Part print with two shaded views. Sizes in mm from the minimum x, y, z corner. A direction names the side the tool comes from. Round coordinates to 2 decimals unless told otherwise and drop trailing zeros. Order: outer loops, then holes, each group sorted by start corner. A loop starts at its lowest first (then second) coordinate and runs counter-clockwise, first axis right, second up. Notation, with made-up numbers: (49, -32.75) -> (66, -32.75) arc R9 ccw to (66, -15.75) -> close; hole circle Ø2 at (7.5, 12). An arc over 180 degrees is marked (long way). Use a Markdown table: item, result. Add a question column.
Item 1: Slice it at C-C, the plane x = 76. Give the cut face in (y, z), plus the area to 3 significant figures.
Item 2: Slice it at A-A, the plane z = 130.5. Give the cut face in (x, y).
Item 3: 3-axis set-ups, long thin cutter, end or side, ignore diameter. For the marked faces 5 and 6: which of +Z, -Z, +X, -X, +Y, -Y reach the whole face in a straight line?
Item 4: Slice it at B-B, the plane y = 154.5. Give the cut face in (x, z), plus the area to 3 significant figures.
Item 5: Two-plate mould, pull along X, no slides. Class the marked faces 1, 2, 3 and 4: released by +X, released by -X, zero draft, split by the parting line, or undercut.
Item 6: Probe L1, parallel to X at y = 129.5, z = 51; L2, parallel to Z at x = 222, y = 11. List the from-to ranges inside material, lowest first.
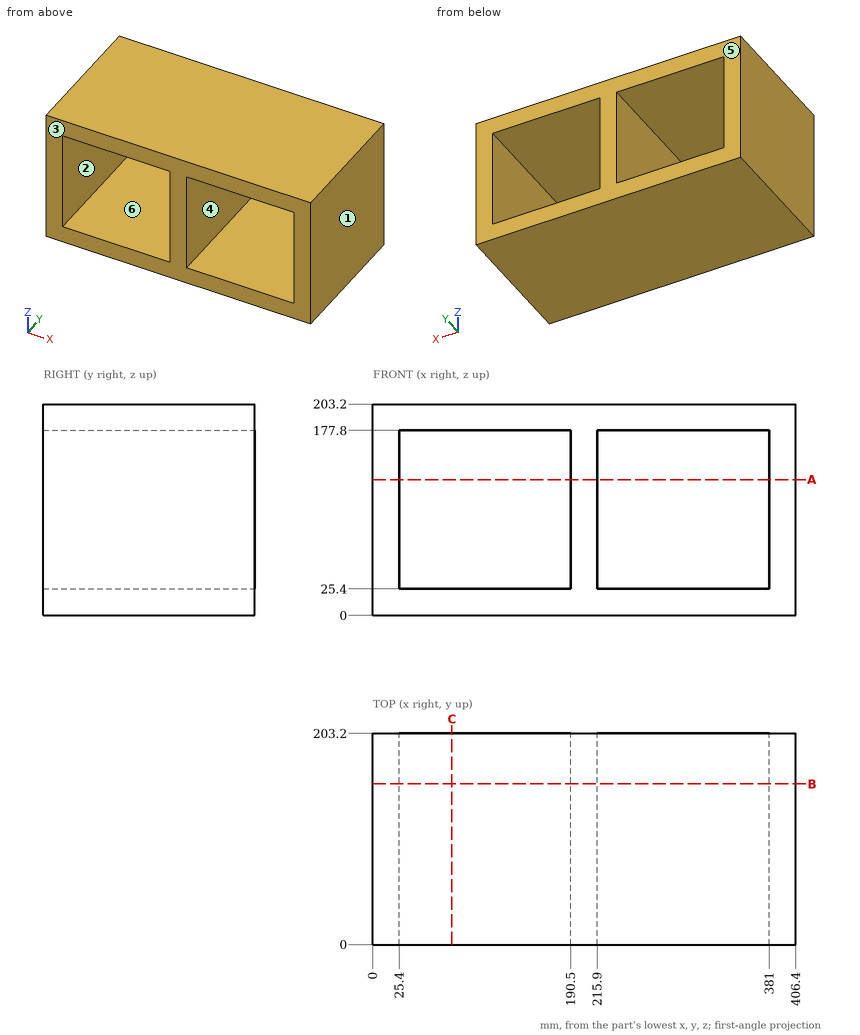
Check sheet entries:
| question | item | result |
|---|---|---|
| 1 | outline | (0, 0) -> (203.2, 0) -> (203.2, 25.4) -> (0, 25.4) -> close; (0, 177.8) -> (203.2, 177.8) -> (203.2, 203.2) -> (0, 203.2) -> close |
| 1 | area | 10,300 mm2 |
| 2 | outline | (0, 0) -> (25.4, 0) -> (25.4, 203.2) -> (0, 203.2) -> close; (190.5, 0) -> (215.9, 0) -> (215.9, 203.2) -> (190.5, 203.2) -> close; (381, 0) -> (406.4, 0) -> (406.4, 203.2) -> (381, 203.2) -> close |
| 3 | face 5 | +Z, -Z, +X, -X, +Y |
| 3 | face 6 | +Y, -Y |
| 4 | outline | (0, 0) -> (406.4, 0) -> (406.4, 203.2) -> (0, 203.2) -> close; hole (25.4, 25.4) -> (190.5, 25.4) -> (190.5, 177.8) -> (25.4, 177.8) -> close; hole (215.9, 25.4) -> (381, 25.4) -> (381, 177.8) -> (215.9, 177.8) -> close |
| 4 | area | 32,300 mm2 |
| 5 | face 1 | released by +X |
| 5 | face 2 | undercut |
| 5 | face 3 | zero draft |
| 5 | face 4 | undercut |
| 6 | L1 | 0 to 25.4, 190.5 to 215.9, 381 to 406.4 |
| 6 | L2 | 0 to 25.4, 177.8 to 203.2 |
